from build123d import *

# Parameters (mm, degrees)
SKETCH1_W           = 24.13
SKETCH1_H           = 17.78
SKETCH1_R           = 2.286
BOSS_EXTRUDE1_DEPTH = 5.08
SKETCH2_R           = 1.778
CUT_EXTRUDE1_DEPTH  = 23.079380086
BOSS_EXTRUDE2_DEPTH = 0.635
LPATTERN1_COUNT     = 10
LPATTERN1_PITCH     = 1.905
SKETCH5_R           = 4.572
CUT_EXTRUDE2_DEPTH  = 1.905
FILLET1_R           = 0.635
FILLET2_R           = 2.54
SKETCH6_R           = 3.81
CUT_EXTRUDE3_DEPTH  = 2.54


with BuildPart() as part:
    # Sketch1 → Boss-Extrude1 (new body)
    with BuildSketch(Plane(origin=(0, 0, 0), x_dir=(1, 0, 0), z_dir=(0, 1, 0))):
        Rectangle(SKETCH1_W, SKETCH1_H)
        with Locations(Location((-7.62, 0, 0), (0, 0, 270))):
            Circle(SKETCH1_R, mode=Mode.SUBTRACT)
        with Locations(Location((7.62, 0, 0), (0, 0, 90))):
            Circle(SKETCH1_R, mode=Mode.SUBTRACT)
    extrude(amount=BOSS_EXTRUDE1_DEPTH)

    # Sketch2 → Cut-Extrude1 (cut, through all)
    with BuildSketch(Plane.XY.offset(8.89)):
        with Locations((0, -0.254)):
            Circle(SKETCH2_R)
    extrude(amount=-CUT_EXTRUDE1_DEPTH, mode=Mode.SUBTRACT)

    # Sketch4 → Boss-Extrude2 (add)
    with BuildSketch(Plane.XY.offset(8.89)):
        with BuildLine():
            ThreePointArc((1.75976362, 0), (0, 1.524), (-1.75976362, 0))
            Line((-1.75976362, 0), (-1.502684265, 0))
            ThreePointArc((-1.502684265, 0), (0, 1.27), (1.502684265, 0))
            Line((1.502684265, 0), (1.75976362, 0))
        make_face()
    boss_extrude2 = extrude(amount=-BOSS_EXTRUDE2_DEPTH)

    # LPattern1: Boss-Extrude2 ×10
    with Locations(*[(0, 0, -i * LPATTERN1_PITCH) for i in range(1, LPATTERN1_COUNT)]):
        add(boss_extrude2)

    # Sketch5 → Cut-Extrude2 (cut)
    with BuildSketch(Plane(origin=(0, 5.08, 0), x_dir=(1, 0, 0), z_dir=(0, 1, 0))):
        with Locations((-7.62, 0)):
            Circle(SKETCH5_R)
        with Locations((7.62, 0)):
            Circle(SKETCH5_R)
    extrude(amount=-CUT_EXTRUDE2_DEPTH, mode=Mode.SUBTRACT)

    # Fillet1
    fillet1_edges = [part.edges().sort_by_distance(p)[0] for p in [
        (12.065, 4.1275, -1.070121021),
        (12.065, 4.1275, 1.070121021),
        (-12.065, 4.1275, 1.070121021),
        (-12.065, 4.1275, -1.070121021),
    ]]
    fillet(fillet1_edges, radius=FILLET1_R)

    # Fillet2
    fillet2_edges = [part.edges().sort_by_distance(p)[0] for p in [
        (-12.065, 2.54, -8.89),
        (12.065, 2.54, -8.89),
        (12.065, 2.54, 8.89),
        (-12.065, 2.54, 8.89),
    ]]
    fillet(fillet2_edges, radius=FILLET2_R)

    # Sketch6 → Cut-Extrude3 (cut, symmetric)
    with BuildSketch(Plane.XY):
        Circle(SKETCH6_R)
    extrude(amount=CUT_EXTRUDE3_DEPTH, both=True, mode=Mode.SUBTRACT)


solid = part.part
Check sheet for the modelled part. Datum: model origin and axes. Units: mm. A direction names the side the tool comes from. Give positions to 0.01 mm unless a question says otherwise; leave off trailing zeros. Write each loop counter-clockwise with the first axis right and the second up, starting at its lowest first coordinate (ties: lowest second). Pieces come first, ordered by that corner, then holes. Notation, with made-up numbers: (31, 40) -> (90, 40) arc R30 ccw to (90, 63) -> close; hole circle Ø4 at (-37, -32). An arc over 180 degrees is marked (long way). Use one line per item in the form item = value. Start each with the question number.
1. Go/stop test with flat-tipped pins: P1, Ø1.7, axis at x = 0, y = 0.5, coming from the +Z side; P2, Ø4.5, axis at x = -7.5, z = -1.5, coming from the +Y side (3 decimals). Record where each tip stops, or that it passes through.
2. Section check A-A (z = 0). Record the cut outline in (x, y) (3 decimals).
3. Mould release check, pull along X, two halves, no side actions. Record for faces 3 (the cylindrical face through (-0.03, 1.27, 4.77)), 4 (the cylindrical face through (-0.03, 1.27, 6.67)), 5 (the flat face through (0, 3, -8.89)), 6 (the flat face through (-12.065, 2, 0)): pulls with the +X half, pulls with the -X half, needs draft (parallel to the pull), parting line crosses it, or undercut.
4. Section check D-D (y = 0.7). Count the separate pieces of the cut face and the enclosed holes in it, and give its area (3 significant figures).
5. Access from +Z, -Z, +X, -X, +Y, -Y to the whole of each face (thin tool, end or side, straight path). Record for faces 1 (the cylindrical face through (0.036, 1.524, -3.801)), 2 (the cylindrical face through (-0.03, 1.27, 2.86)).
6. Section check B-B (x = 7.62). Record the cut outline in (y, z) (3 decimals).
7. Thickness scan on line 1 along Z through (x, y) = (7.62, 4); line 2 along X through (y, z) = (1.95, 0) (3 decimals); line 3 along Z through (x, y) = (3.25, 1.8). Record the ranges inside material, lowest first. Write a range as from..to.
Conclusion:
q1.P1 = 8.89
q1.P2 = 3.175
q2.outline = (-12.065, 0) -> (-9.906, 0) -> (-9.906, 3.175) -> (-12.065, 3.175) -> close; (-5.334, 0) -> (-3.81, 0) arc R3.81 cw to (3.81, 0) -> (5.334, 0) -> (5.334, 3.175) -> (3.048, 3.175) -> (3.048, 5.08) -> (-3.048, 5.08) -> (-3.048, 3.175) -> (-5.334, 3.175) -> close; (9.906, 0) -> (12.065, 0) -> (12.065, 3.175) -> (9.906, 3.175) -> close
q3.face_3 = undercut
q3.face_4 = undercut
q3.face_5 = needs draft
q3.face_6 = pulls with the -X half
q4.separate_pieces = 2
q4.enclosed_holes = 2
q4.area = 318 mm²
q5.face_1 = -Y
q5.face_2 = +Z, -Z, -Y
q6.outline = (0, -8.89) -> (5.08, -8.89) -> (5.08, -4.572) -> (3.175, -4.572) -> (3.175, -2.286) -> (0, -2.286) -> close; (0, 2.286) -> (3.175, 2.286) -> (3.175, 4.572) -> (5.08, 4.572) -> (5.08, 8.89) -> (0, 8.89) -> close
q7.line_1 = -8.89..-4.57, 4.57..8.89
q7.line_2 = -12.065..-9.906, -5.334..-3.273, 3.273..5.334, 9.906..12.065
q7.line_3 = -8.89..-2.54, 2.54..8.89
